Read the model definition and answer for the solid it produces. Units are mm, in the model's axes. Give positions to 0.01 mm unless a question says otherwise; leave off trailing zeros. Order: outer loops, then holes, each group sorted by start corner. A loop starts at its lowest first (then second) coordinate and runs counter-clockwise, first axis right, second up. Notation, with made-up numbers: (-37.75, 28) -> (-31.75, 28) arc R18 ccw to (-31.75, 51) -> close; hole circle Ø9 at (-2.5, -7). An arc over 180 degrees is marked (long way). Use one line per item in the form item = value.
```python
from build123d import *

# Parameters (mm, degrees)
F1_DEPTH     = 1.5
F3_DEPTH     = 10.5
F4_T4_DEPTH  = 31
F4_T9_ANGLE  = 180
F4_T14_DEPTH = 31
F4_T19_ANGLE = 180
F5_T         = 2.5
F5_T3_DEPTH  = 36
F5_T6_ANGLE  = 180.000000001
F5_T8_ANGLE  = 180.000000001
F6_R         = 2


# Not quite as in the source:
# - a fillet or chamfer that OpenCascade refuses, or shapes differently, is made with other operations: its cross-section is extruded or revolved along the edge and cut away or added
# - a shell that OpenCascade refuses in one call is made with other operations: the cavity is built on its own and cut out


with BuildPart() as f1:
    # F0 (on Top) → F1 (new body)
    with BuildSketch(Plane.XY):
        with BuildLine():
            Line((15.5, 9.5), (-15.5, 9.5))
            ThreePointArc((-15.5, 9.5), (-25, 0), (-15.5, -9.5))
            Line((-15.5, -9.5), (15.5, -9.5))
            ThreePointArc((15.5, -9.5), (25, 0), (15.5, 9.5))
        make_face()
        with BuildLine():
            ThreePointArc((-15.5, -8), (-23.5, 0), (-15.5, 8))
            Line((-15.5, 8), (15.5, 8))
            ThreePointArc((15.5, 8), (23.5, 0), (15.5, -8))
            Line((15.5, -8), (-15.5, -8))
        make_face(mode=Mode.SUBTRACT)
        with BuildLine():
            Line((15.5, 8), (-15.5, 8))
            ThreePointArc((-15.5, 8), (-23.5, 0), (-15.5, -8))
            Line((-15.5, -8), (15.5, -8))
            ThreePointArc((15.5, -8), (23.5, 0), (15.5, 8))
        make_face()
    extrude(amount=-F1_DEPTH)

    # F2 (on face) → F3 (join)
    with BuildSketch(Plane.XY):
        with BuildLine():
            Line((15.5, 8), (-15.5, 8))
            ThreePointArc((-15.5, 8), (-23.5, 0), (-15.5, -8))
            Line((-15.5, -8), (15.5, -8))
            ThreePointArc((15.5, -8), (23.5, 0), (15.5, 8))
        make_face()
    extrude(amount=F3_DEPTH)

    # F4: chamfer of 3 x 11.1961524227 on 4 edges, made by hand


with BuildPart() as f4_tool2:
    # F4_s3 → F4_t4 (new body)
    with BuildSketch(Plane.YZ.offset(-15.5)):
        Polygon((-8, -0.6961524227), (-5, 10.5), (-8, 10.5), align=None)
    extrude(amount=F4_T4_DEPTH)

    split(bisect_by=Plane.XY, keep=Keep.TOP)


with BuildPart() as f1_1:
    add(f1.part)

    # F4_t1: cut F4_tool2
    add(f4_tool2.part, mode=Mode.SUBTRACT)


with BuildPart() as f4_tool7:
    # F4_s8 → F4_t9 (revolve)
    with BuildSketch(Plane.YZ.offset(15.5)):
        Polygon((-8, -0.6961524227), (-5, 10.5), (-8, 10.5), align=None)
    revolve(axis=Axis((15.5, 0, 10.5), (0, 0, 1)), revolution_arc=F4_T9_ANGLE)

    split(bisect_by=Plane.XY, keep=Keep.TOP)


with BuildPart() as f1_2:
    add(f1_1.part)

    # F4_t6: cut F4_tool7
    add(f4_tool7.part, mode=Mode.SUBTRACT)


with BuildPart() as f4_tool12:
    # F4_s13 → F4_t14 (new body)
    with BuildSketch(Plane.YZ.offset(15.5)):
        Polygon((8, -0.6961524227), (5, 10.5), (8, 10.5), align=None)
    extrude(amount=-F4_T14_DEPTH)

    split(bisect_by=Plane.XY, keep=Keep.TOP)


with BuildPart() as f1_3:
    add(f1_2.part)

    # F4_t11: cut F4_tool12
    add(f4_tool12.part, mode=Mode.SUBTRACT)


with BuildPart() as f4_tool17:
    # F4_s18 → F4_t19 (revolve)
    with BuildSketch(Plane.YZ.offset(-15.5)):
        Polygon((8, -0.6961524227), (5, 10.5), (8, 10.5), align=None)
    revolve(axis=Axis((-15.5, 0, 10.5), (0, 0, 1)), revolution_arc=F4_T19_ANGLE)

    split(bisect_by=Plane.XY, keep=Keep.TOP)


with BuildPart() as f1_4:
    add(f1_3.part)

    # F4_t16: cut F4_tool17
    add(f4_tool17.part, mode=Mode.SUBTRACT)

    # F5: shell of thickness 2.5, made by hand


with BuildPart() as f5_core1:
    # F5_t2: copy of F1
    add(f1_4.part)

    # the walls: a layer under each face that stays
    f5_faces = [f5_core1.faces().sort_by_distance(p)[0] for p in [
        (25, 0, -0.75),
        (0, -9.5, -0.75),
        (0, 9.5, -0.75),
        (-21.4285714286, -5.4285714286, 0),
        (-25, 0, -0.75),
        (0, -6.4067332603, 5.25),
        (0, 6.4067332603, 5.25),
        (21.9067332603, 0, 5.25),
        (-21.9067332603, 0, 5.25),
        (0, 0, 10.5),
    ]]
    thicken(f5_faces, amount=-F5_T, mode=Mode.SUBTRACT)

    # F5_s4 → F5_t3 (cut)
    with BuildSketch(Plane.YZ.offset(-18)):
        Polygon((-7.8376146662, 0.0314704761), (-7.8134665205, -2.5), (-5.8951490506, -2.5), (-5.3986519548, -0.6470476128), align=None)
        Polygon((7.8376146662, 0.0314704761), (7.8134665205, -2.5), (5.8951490506, -2.5), (5.3986519548, -0.6470476128), align=None)
    extrude(amount=F5_T3_DEPTH, mode=Mode.SUBTRACT)

    # F5_s5 → F5_t6 (revolve, cut)
    with BuildSketch(Plane.YZ.offset(-15.5)):
        Polygon((7.8376146662, 0.0314704761), (7.8134665205, -2.5), (5.8951490506, -2.5), (5.3986519548, -0.6470476128), align=None)
    revolve(axis=Axis((-15.5, 0, 0), (0, 0, 1)), revolution_arc=F5_T6_ANGLE, mode=Mode.SUBTRACT)

    # F5_s7 → F5_t8 (revolve, cut)
    with BuildSketch(Plane.YZ.offset(15.5)):
        Polygon((-7.8376146662, 0.0314704761), (-7.8134665205, -2.5), (-5.8951490506, -2.5), (-5.3986519548, -0.6470476128), align=None)
    revolve(axis=Axis((15.5, 0, 0), (0, 0, 1)), revolution_arc=F5_T8_ANGLE, mode=Mode.SUBTRACT)


with BuildPart() as f1_5:
    add(f1_4.part)

    # what is left inside the walls is the cavity
    f5_cavity = [f5_core1.part.solids().sort_by_distance(p)[0] for p in [
        (0, -1.875733, -1.475),
    ]]
    add(f5_cavity, mode=Mode.SUBTRACT)

    # F6
    f6_edges = [f1_5.edges().sort_by_distance(p)[0] for p in [
        (-20.5, 0, 10.5),
    ]]
    fillet(f6_edges, radius=F6_R)


solid = f1_5.part
```
Item 1: The part is cut by section C-C on z = 1. Give the vertices of the cut face in (x, y).
Checks:
outline = (-15.5, -7.55) -> (15.5, -7.55) arc R7.55 ccw to (15.5, 7.55) -> (-15.5, 7.55) arc R7.55 ccw to start; hole (-15.5, -4.96) -> (15.5, -4.96) arc R4.96 ccw to (15.5, 4.96) -> (-15.5, 4.96) arc R4.96 ccw to start
Item 2: Given pin 1 Ø1 at (y, z) = (3, 5.5) entering from -X; pin 2 Ø1 at (x, z) = (-11.5, 5.5) entering from +Y; pin 3 Ø5 at (x, y) = (-7.5, 0) entering from -Z, each flat-ended and moving along its own axis, determine where each tip first touches the part or whether it passes through.
Checks:
pin_1 = -21.37
pin_2 = 6.47
pin_3 = 8
Item 3: The part is cut by section B-B on z = 3.25. Give the vertices of the cut face in (x, y), and give its area (3 significant figures).
Checks:
outline = (-15.5, -6.94) -> (15.5, -6.94) arc R6.94 ccw to (15.5, 6.94) -> (-15.5, 6.94) arc R6.94 ccw to start; hole (-15.5, -4.35) -> (15.5, -4.35) arc R4.35 ccw to (15.5, 4.35) -> (-15.5, 4.35) arc R4.35 ccw to start
area = 252 mm²
Item 4: The part is cut by section A-A on x = 10.5. Give the vertices of the cut face in (y, z).
Checks:
outline = (-9.5, -1.5) -> (-5.63, -1.5) -> (-3.08, 8) -> (3.08, 8) -> (5.63, -1.5) -> (9.5, -1.5) -> (9.5, 0) -> (7.81, 0) -> (5.4, 9.02) arc R2 ccw to (3.47, 10.5) -> (-3.47, 10.5) arc R2 ccw to (-5.4, 9.02) -> (-7.81, 0) -> (-9.5, 0) -> close
Item 5: Straight lines are drawn through the part: L1, parallel to Z at x = -15, y = 3; L2, parallel to Z at x = 20.5, y = 6.25; L3, parallel to X at y = 1.5, z = 4.5. For each, find the intervals that lie inside material, in ascending order. Write a range as from..to.
Checks:
L1 = 8..10.5
L2 = -1.5..0
L3 = -21.94..-19.23, 19.23..21.94
Item 6: Determine the mould class of faces 1 (the cylindrical face through (-25, 0, -1)), 2 (the cylindrical face through (25, 0, -1)), 3 (the flat face through (2, 8, 0)), 4 (the flat face through (0, 0, 8)) for opening direction X: +X half, -X half, draft (parallel to the pull), parting line (faces both ways), or undercut.
Checks:
face_1 = -X half
face_2 = +X half
face_3 = draft
face_4 = undercut
